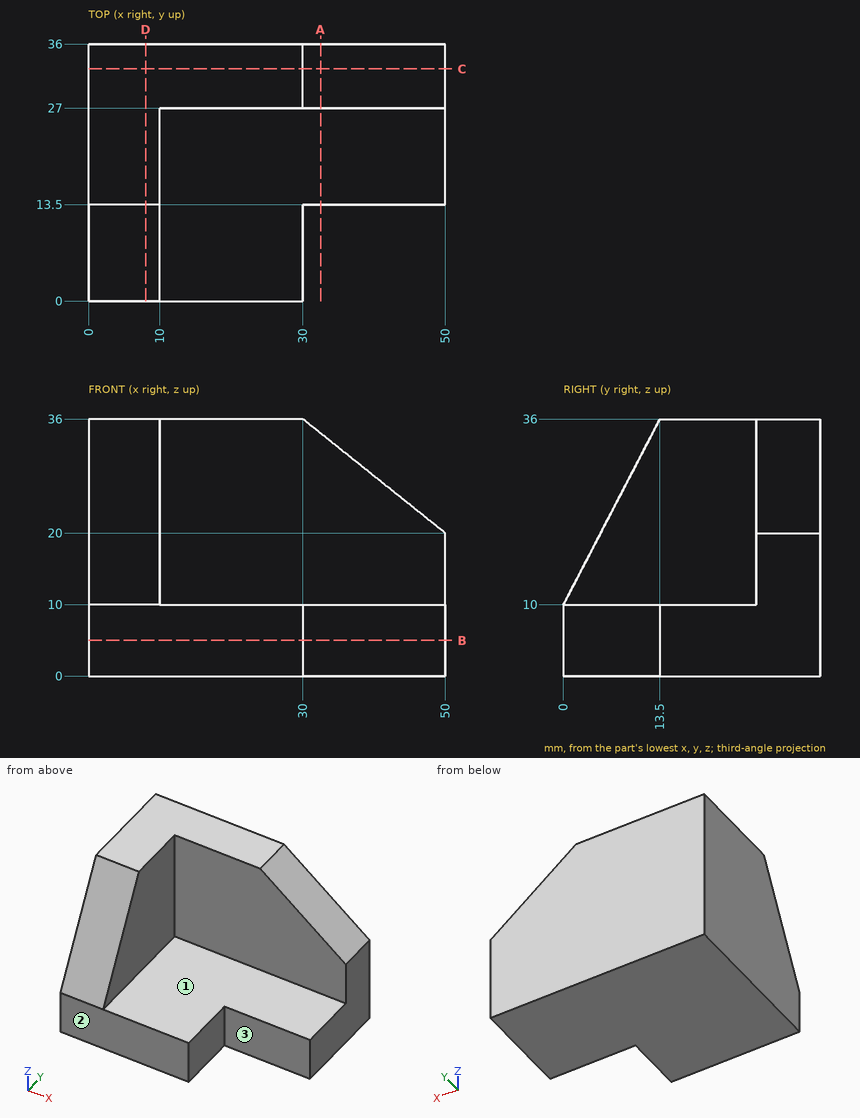
Geometry: see drawing. Coordinates: mm, zero at the bounding-box minimum. A direction names the side the tool comes from. Give positions to 0.01 mm unless a question says otherwise; leave off trailing zeros. Order: outer loops, then holes, each group sorted by start corner. A loop starts at its lowest first (then second) coordinate and runs counter-clockwise, first axis right, second up. Notation, with made-up numbers: (-1.75, 34.25) - (56.25, 34.25) arc R31 ccw to (56.25, 58.25) - close; hole circle Ø10 at (-7, -31). An arc over 180 degrees is marked (long way). Use a Markdown table: item, result.
(1) Section query B-B (z = 5). Output: boundary loops of the cut face in (x, y).
Computed values:
| item | result |
|---|---|
| outline | (0, 0) - (30, 0) - (30, 13.5) - (50, 13.5) - (50, 36) - (0, 36) - close |
(2) Section query A-A (x = 32.5). Output: boundary loops of the cut face in (y, z).
Computed values:
| item | result |
|---|---|
| outline | (13.5, 0) - (36, 0) - (36, 34) - (27, 34) - (27, 10) - (13.5, 10) - close |
(3) Section query D-D (x = 8). Output: boundary loops of the cut face in (y, z).
Computed values:
| item | result |
|---|---|
| outline | (0, 0) - (36, 0) - (36, 36) - (13.5, 36) - (0, 10) - close |
(4) Pin query (flat end, axial travel): pin 1 (5 mm diameter, centred on x = 9.5, z = 14.5, fed in from -Y); pin 2 (8 mm diameter, centred on y = 30.5, z = 25, fed in from +X); pin 3 (3 mm diameter, centred on x = 42, z = 4.5, fed in from -Y). Return the tip coordinate at first contact, or that it passes through.
Computed values:
| item | result |
|---|---|
| pin 1 | stops at y = 1.04 |
| pin 2 | stops at x = 48.75 |
| pin 3 | stops at y = 13.5 |
(5) Line query: line 1 (X direction, y = 17, z = 28); line 2 (Y direction, x = 24, z = 31). Output: solid intervals per line, ascending. Write a range as from..to.
Computed values:
| item | result |
|---|---|
| line 1 | x = 0..10 |
| line 2 | y = 27..36 |
(6) Access query for the marked faces 1, 2 and 3. Directions: +Z, -Z, +X, -X, +Y, -Y. A direction counts if a zero-diameter tool reaches every point of the face in a straight line with its end or side. Return the directions, or none.
Computed values:
| item | result |
|---|---|
| face 1 | +Z, +X, -Y |
| face 2 | +Z, -Z, +X, -X, -Y |
| face 3 | +Z, -Z, +X, -Y |
(7) Section query C-C (y = 32.5). Output: boundary loops of the cut face in (x, z).
Computed values:
| item | result |
|---|---|
| outline | (0, 0) - (50, 0) - (50, 20) - (30, 36) - (0, 36) - close |
